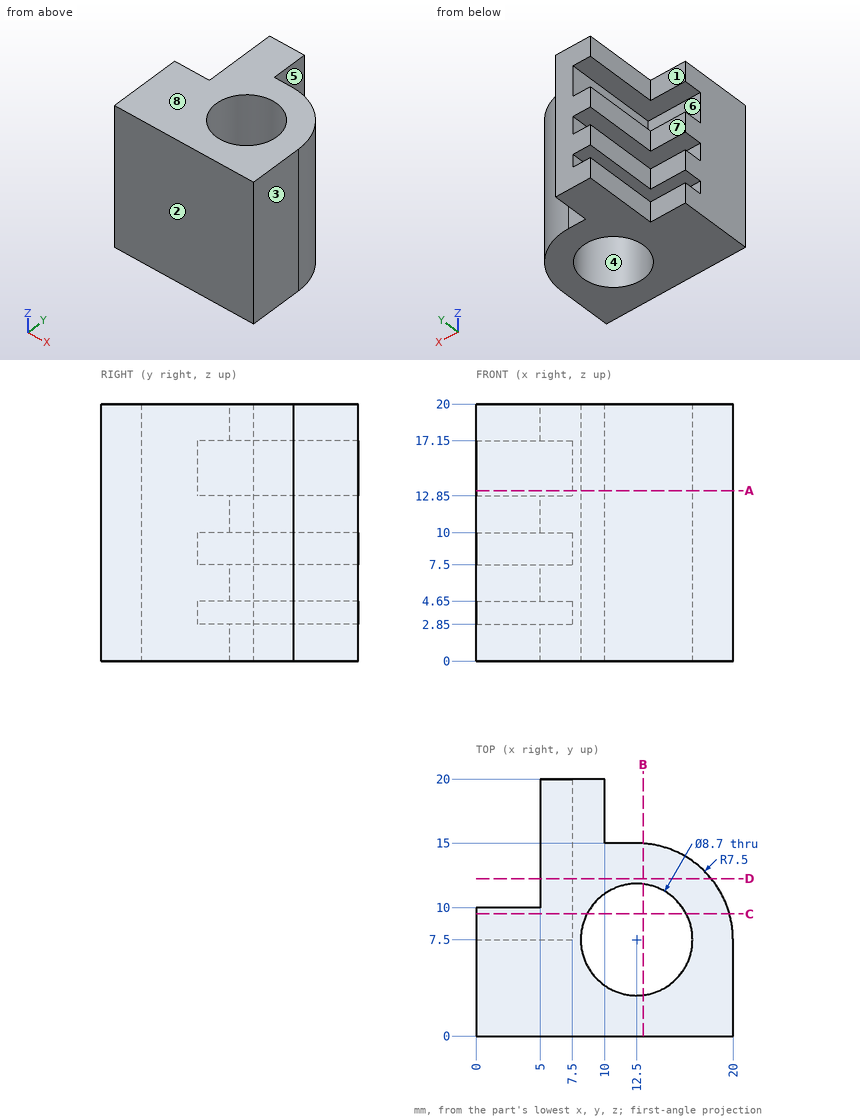
Study the drawing (mm; zero at the part's minimum x, y, z) and answer. A direction names the side the tool comes from. Give positions to 0.01 mm unless a question says otherwise; leave off trailing zeros. Order: outer loops, then holes, each group sorted by start corner. A loop starts at its lowest first (then second) coordinate and runs counter-clockwise, first axis right, second up.
1. The mould has two halves that part along Y. Classify the marked faces 1, 2, 3 and 4: released by +Y, released by -Y, zero draft, split by the parting line, or undercut.
Result sheet:
face 1: released by +Y
face 2: released by -Y
face 3: zero draft
face 4: undercut
2. For the marked faces 5, 6, 7 and 8, determine the directions among +Z, -Z, +X, -X, +Y, -Y from which every point of the face is accessible in a straight line to the end or side of a thin tool.
Result sheet:
face 5: +Z, -Z, +X, +Y
face 6: -X, +Y
face 7: +Z, -Z, -X, +Y
face 8: +Z, +X, -X, +Y, -Y
3. Straight lines are drawn through the part: L1, parallel to Z at x = 4.5, y = 7.75; L2, parallel to Y at x = 12.5, z = 9; L3, parallel to Y at x = 5, z = 16. For each, find the intervals that lie inside material, in ascending order.
Result sheet:
L1: z = 0 to 2.85, 4.65 to 7.5, 10 to 12.85, 17.15 to 20
L2: y = 0 to 3.15, 11.85 to 15
L3: y = 0 to 7.5
4. Each of these flat-tipped pins is pushed along its axis until it touches: P1, Ø2.5, axis at x = 1.5, z = 6, coming from the +Y side; P2, Ø10, axis at x = 15.5, z = 7, coming from the +Y side; P3, Ø2.5, axis at y = 14, z = 11, coming from the -X side; P4, Ø10, axis at x = 3, z = 5, coming from the +Y side. Where does it stop, or does it pass through?
Result sheet:
P1: stops at y = 10
P2: stops at y = 15
P3: stops at x = 5
P4: stops at y = 20
5. Section D-D, the plane y = 12.25 is taken. Determine the outline of the cut face in (x, z).
Result sheet:
outline: (5, 0) - (18.3, 0) - (18.3, 20) - (5, 20) - (5, 17.15) - (7.5, 17.15) - (7.5, 12.85) - (5, 12.85) - (5, 10) - (7.5, 10) - (7.5, 7.5) - (5, 7.5) - (5, 4.65) - (7.5, 4.65) - (7.5, 2.85) - (5, 2.85) - close
6. Section C-C, the plane y = 9.5 is taken. Determine the outline of the cut face in (x, z).
Result sheet:
outline: (0, 0) - (8.64, 0) - (8.64, 20) - (0, 20) - (0, 17.15) - (7.5, 17.15) - (7.5, 12.85) - (0, 12.85) - (0, 10) - (7.5, 10) - (7.5, 7.5) - (0, 7.5) - (0, 4.65) - (7.5, 4.65) - (7.5, 2.85) - (0, 2.85) - close; (16.36, 0) - (19.73, 0) - (19.73, 20) - (16.36, 20) - close
7. Section B-B, the plane x = 13 is taken. Determine the outline of the cut face in (y, z).
Result sheet:
outline: (0, 0) - (3.18, 0) - (3.18, 20) - (0, 20) - close; (11.82, 0) - (14.98, 0) - (14.98, 20) - (11.82, 20) - close
8. Section A-A, the plane z = 13.25 is taken. Determine the outline of the cut face in (x, y).
Result sheet:
outline: (0, 0) - (20, 0) - (20, 7.5) arc R7.5 ccw to (12.5, 15) - (10, 15) - (10, 20) - (7.5, 20) - (7.5, 7.5) - (0, 7.5) - close; hole circle Ø8.7 at (12.5, 7.5)
